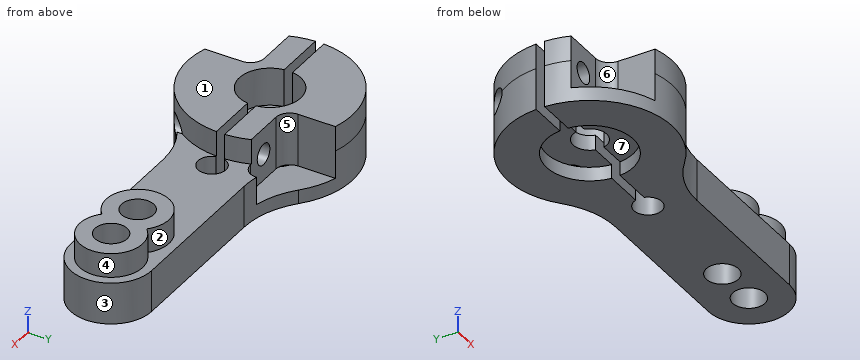
```python
from build123d import *

# Parameters (mm, degrees)
SKETCH1_R           = 1.4605
SKETCH1_R_2         = 1.524
SKETCH1_R_3         = 1.27
BOSS_EXTRUDE2_DEPTH = 3.81
SKETCH2_R           = 1.4605
BOSS_EXTRUDE3_DEPTH = 2.2098
SKETCH3_R           = 7.493
SKETCH3_R_2         = 2.794
BOSS_EXTRUDE4_DEPTH = 2.286
SKETCH4_R           = 2.794
CUT_EXTRUDE1_DEPTH  = 3.4544
CUT_EXTRUDE2_DEPTH  = 4.826
SKETCH6_R           = 0.9525
CUT_EXTRUDE3_DEPTH  = 11.033
SKETCH7_R           = 0.9525
CUT_EXTRUDE4_DEPTH  = 11.0330001
SKETCH8_W           = 15.900663219
SKETCH8_H           = 0.762
CUT_EXTRUDE5_DEPTH  = 7.0960001
SKETCH9_R           = 3.937
CUT_EXTRUDE6_DEPTH  = 1.27


with BuildPart() as part:
    # Sketch1 → Boss-Extrude2 (new body)
    with BuildSketch(Plane.XY):
        with BuildLine():
            Line((24, 3.683), (10.03219617, 3.683))
            ThreePointArc((10.03219617, 3.683), (7.326823365, 4.179422389), (4.973946, 5.604008403))
            ThreePointArc((4.973946, 5.604008403), (-7.493, 0), (4.973946, -5.604008403))
            ThreePointArc((4.973946, -5.604008403), (7.326823365, -4.179422389), (10.03219617, -3.683))
            Line((10.03219617, -3.683), (24, -3.683))
            ThreePointArc((24, -3.683), (27.683, 0), (24, 3.683))
        make_face()
        with Locations((24, 0)):
            Circle(SKETCH1_R, mode=Mode.SUBTRACT)
        with Locations((20, 0)):
            Circle(SKETCH1_R, mode=Mode.SUBTRACT)
        Circle(SKETCH1_R_2, mode=Mode.SUBTRACT)
        with Locations((8.763, 0)):
            Circle(SKETCH1_R_3, mode=Mode.SUBTRACT)
    extrude(amount=BOSS_EXTRUDE2_DEPTH)

    # Sketch2 → Boss-Extrude3 (add)
    with BuildSketch(Plane.XY.offset(3.81)):
        with BuildLine():
            ThreePointArc((22, -2.040908192), (26.8575, 0), (22, 2.040908192))
            ThreePointArc((22, 2.040908192), (17.1425, 0), (22, -2.040908192))
        make_face()
        with Locations((20, 0)):
            Circle(SKETCH2_R, mode=Mode.SUBTRACT)
        with Locations((24, 0)):
            Circle(SKETCH2_R, mode=Mode.SUBTRACT)
    extrude(amount=BOSS_EXTRUDE3_DEPTH)

    # Sketch3 → Boss-Extrude4 (add)
    with BuildSketch(Plane.XY.offset(3.81)):
        Circle(SKETCH3_R)
        Circle(SKETCH3_R_2, mode=Mode.SUBTRACT)
    extrude(amount=BOSS_EXTRUDE4_DEPTH)

    # Sketch4 → Cut-Extrude1 (cut)
    with BuildSketch(Plane.XY.offset(6.096)):
        Circle(SKETCH4_R)
    extrude(amount=-CUT_EXTRUDE1_DEPTH, mode=Mode.SUBTRACT)

    # Sketch5 → Cut-Extrude2 (cut)
    with BuildSketch(Plane.XY.offset(6.096)):
        with BuildLine():
            Line((-2.090104165, -8.640089248), (-2.090104165, -3.81))
            ThreePointArc((-2.090104165, -3.81), (-2.462078553, -2.911974388), (-3.360104165, -2.54))
            Line((-3.360104165, -2.54), (-7.170104165, -2.54))
            ThreePointArc((-7.170104165, -2.54), (-8.068129777, -2.911974388), (-8.440104165, -3.81))
            Line((-8.440104165, -3.81), (-8.440104165, -8.640089248))
            Line((-8.440104165, -8.640089248), (-2.090104165, -8.640089248))
        make_face()
        with BuildLine():
            Line((8.440104165, 8.640089248), (2.090104165, 8.640089248))
            Line((2.090104165, 8.640089248), (2.090104165, 3.81))
            ThreePointArc((2.090104165, 3.81), (2.462078553, 2.911974388), (3.360104165, 2.54))
            Line((3.360104165, 2.54), (7.170104165, 2.54))
            ThreePointArc((7.170104165, 2.54), (8.068129777, 2.911974388), (8.440104165, 3.81))
            Line((8.440104165, 3.81), (8.440104165, 8.640089248))
        make_face()
    extrude(amount=-CUT_EXTRUDE2_DEPTH, mode=Mode.SUBTRACT)

    # Sketch6 → Cut-Extrude3 (cut, through all)
    with BuildSketch(Plane(origin=(0, -2.54, 0), x_dir=(-1, 0, 0), z_dir=(0, -1, 0))):
        with Locations((5.20473111, -3.683)):
            Circle(SKETCH6_R)
    extrude(amount=-CUT_EXTRUDE3_DEPTH, mode=Mode.SUBTRACT)

    # Sketch7 → Cut-Extrude4 (cut, through all)
    with BuildSketch(Plane(origin=(0, 2.54, 0), x_dir=(1, 0, 0), z_dir=(0, 1, 0))):
        with Locations((5.20473111, -3.683)):
            Circle(SKETCH7_R)
    extrude(amount=-CUT_EXTRUDE4_DEPTH, mode=Mode.SUBTRACT)

    # Sketch8 → Cut-Extrude5 (cut, through all)
    with BuildSketch(Plane.XY.offset(6.096)):
        with Locations((0.457331609, 0)):
            Rectangle(SKETCH8_W, SKETCH8_H)
    extrude(amount=-CUT_EXTRUDE5_DEPTH, mode=Mode.SUBTRACT)

    # Sketch9 → Cut-Extrude6 (cut)
    with BuildSketch(Plane(origin=(0, 0, 0), x_dir=(-1, 0, 0), z_dir=(0, 0, -1))):
        Circle(SKETCH9_R)
    extrude(amount=-CUT_EXTRUDE6_DEPTH, mode=Mode.SUBTRACT)


solid = part.part
```
Can you work these out from the model? Positions are in its coordinate system, mm. Face numbers are marked on the shaded views. A direction names the side the tool comes from. Coordinates: 2 decimals unless noted, no trailing zeros. Loops run counter-clockwise (first coordinate to the right, second up) from the corner with the lowest first, then second, coordinate; pieces in that order, holes last. Notation, with made-up numbers: (-6, 57) -> (33, 57) arc R27 ccw to (33, 93) -> close; hole circle Ø7 at (-32.75, 45). An arc over 180 degrees is marked (long way). Answer as a JSON object with one key per item and string values.
1) For the marked faces 4, 5, 6 and 7, which set-ups out of +Z, -Z, +X, -X, +Y, -Y let a thin tool reach every point of the face, with its end or its side?
Results:
{"face 4": "+Z", "face 5": "+Z, +Y", "face 6": "+Z, -X, -Y", "face 7": "-Z"}
2) Imagine slicing it at D-D (z = 5.5). Please give me the cut outline in (x, y) (1 decimal), then the cut area to 3 significant figures.
Results:
{"outline": "(-7.5, -0.4) arc R7.5 ccw to (-7, -2.5) -> (-3.4, -2.5) arc R1.3 cw to (-2.1, -3.8) -> (-2.1, -7.2) arc R7.5 ccw to (7.5, -0.4) -> (2.8, -0.4) arc R2.8 cw to (-2.8, -0.4) -> close; (-7.5, 0.4) -> (-2.8, 0.4) arc R2.8 cw to (2.8, 0.4) -> (7.5, 0.4) arc R7.5 ccw to (7, 2.5) -> (3.4, 2.5) arc R1.3 cw to (2.1, 3.8) -> (2.1, 7.2) arc R7.5 ccw to start; (22, -2) arc R2.9 ccw (long way) to (22, 2) arc R2.9 ccw (long way) to start; hole circle Ø2.9 at (20, 0); hole circle Ø2.9 at (24, 0)", "area": "148 mm^2"}
3) Imagine slicing it at B-B (x = 20). Please give me the cut outline in (y, z).
Results:
{"outline": "(-3.68, 0) -> (-1.46, 0) -> (-1.46, 6.02) -> (-2.86, 6.02) -> (-2.86, 3.81) -> (-3.68, 3.81) -> close; (1.46, 0) -> (3.68, 0) -> (3.68, 3.81) -> (2.86, 3.81) -> (2.86, 6.02) -> (1.46, 6.02) -> close"}
4) For P1, Ø1.8, axis at x = -5, z = 3, coming from the +Y side; P2, Ø0.7, axis at x = -0.5, y = 1.5, coming from the +Z side; P3, Ø1.8, axis at x = -4, z = 4.5, coming from the -Y side, each with a flat end and sliding along its axis, tell me the tip position at first contact or that it passes through.
Results:
{"P1": "stops at y = 6.27", "P2": "stops at z = 2.64", "P3": "stops at y = -2.57"}
5) Imagine slicing it at C-C (z = 2.25). Please give me the cut outline in (x, y).
Results:
{"outline": "(-7.48, -0.38) arc R7.49 ccw to (-7.05, -2.54) -> (-3.36, -2.54) arc R1.27 cw to (-2.09, -3.81) -> (-2.09, -7.2) arc R7.49 ccw to (4.97, -5.6) arc R7.62 cw to (10.03, -3.68) -> (24, -3.68) arc R3.68 ccw to (24, 3.68) -> (10.03, 3.68) arc R7.62 cw to (8.44, 3.85) -> (8.44, 3.81) arc R1.27 cw to (7.17, 2.54) -> (3.36, 2.54) arc R1.27 cw to (2.09, 3.81) -> (2.09, 7.2) arc R7.49 ccw to (-7.48, 0.38) -> (-1.48, 0.38) arc R1.52 cw to (1.48, 0.38) -> (7.55, 0.38) arc R1.27 cw (long way) to (7.55, -0.38) -> (1.48, -0.38) arc R1.52 cw to (-1.48, -0.38) -> close; hole circle Ø2.92 at (20, 0); hole circle Ø2.92 at (24, 0)"}
6) Imagine slicing it at A-A (y = 0). Please give me the cut outline in (x, z).
Results:
{"outline": "(10.03, 0) -> (18.54, 0) -> (18.54, 6.02) -> (17.14, 6.02) -> (17.14, 3.81) -> (10.03, 3.81) -> close; (21.46, 0) -> (22.54, 0) -> (22.54, 6.02) -> (21.46, 6.02) -> close; (25.46, 0) -> (27.68, 0) -> (27.68, 3.81) -> (26.86, 3.81) -> (26.86, 6.02) -> (25.46, 6.02) -> close"}
7) Thinking about a two-plate mould opening in X: for the marked faces 1, 2 and 3, which applies, pulls with the +X half, pulls with the -X half, needs draft (parallel to the pull), parting line crosses it, or undercut?
Results:
{"face 1": "needs draft", "face 2": "undercut", "face 3": "pulls with the +X half"}
8) If I drill on line 1 (Y direction, x = 15, z = 1.25); line 2 (Y direction, x = 5, z = 0.75); line 3 (Z direction, x = 22.5, y = 0.5), over which ranges is the centre line in solid material (lowest first)?
Results:
{"line 1": "y = -3.68 to 3.68", "line 2": "y = -5.58 to -0.38, 0.38 to 5.58", "line 3": "z = 0 to 6.02"}
